Could you check a few things on this model? Use its own coordinates, in mm. Face numbers are marked on the shaded views. A direction names the side the tool comes from. Coordinates: 2 decimals unless noted, no trailing zeros. Order: outer loops, then holes, each group sorted by start corner. A loop starts at its lowest first (then second) coordinate and runs counter-clockwise, first axis right, second up. Notation, with made-up numbers: (6.25, 63) -> (41.25, 63) arc R25 ccw to (41.25, 101) -> close; hole circle Ø8 at (3.5, 87). An arc over 180 degrees is marked (long way). Use a Markdown table: item, result. Add a question column.
1) Thinking about a two-plate mould opening in Z: for the marked faces 1, 2 and 3, which applies, +Z half, -Z half, draft (parallel to the pull), parting line (faces both ways), or undercut?
2) If I drill on L1, parallel to Y at x = 5.5, z = -1; L2, parallel to Z at x = -2.5, y = 0.5; L3, parallel to X at y = 3.15, z = -18.5, over which ranges is the centre line in solid material (lowest first)? Write a range as [from, to].
3) If we section it at D-D (x = 5): Write out the boundary of the cut face in (y, z).
4) Which directions (+Z, -Z, +X, -X, +Y, -Y) give clear straight access to the entire face, cutting with the end or side of a thin tool? Please do the marked faces 4, 5 and 6.
5) If we section it at C-C (y = 3.3): Write out the boundary of the cut face in (x, z).
6) Will these pins go through, and if not, where does the flat tip stop? pin 1 Ø2 at (x, z) = (-1.5, -2.5) entering from +Y; pin 2 Ø6 at (x, z) = (4.5, -13) entering from +Y; pin 3 Ø1.5 at (x, y) = (1.5, 2.5) entering from +Z.
```python
from build123d import *

# Parameters (mm, degrees)
SM_BASE_FLANGE_1_DEPTH = 0.1
SKETCH_6_W             = 12.5
SKETCH_6_H             = 4
EXTRUDE_1_DEPTH        = 0.1
SKETCH_7_W             = 8.5
SKETCH_7_H             = 8.5
EXTRUDE_2_DEPTH        = 0.1
SKETCH_8_W             = 8.5
SKETCH_8_H             = 8.5
EXTRUDE_3_DEPTH        = 5.07
SKETCH_9_R             = 3
CUT_EXTRUDE_1_DEPTH    = 0.2
FILLET_2_R             = 0.5
FILLET_3_R             = 0.2
SKETCH_11_R            = 0.25
SKETCH_11_W            = 0.4
SKETCH_11_H            = 0.1
SKETCH_11_W_2          = 0.428641975
CUT_EXTRUDE_2_DEPTH    = 0.05
FILLET_4_R             = 0.2
FILLET_5_R             = 0.2
SKETCH_13_R            = 0.75
CUT_EXTRUDE_3_DEPTH    = 0.05
DOME_1_FACE_RADIUS     = 0.75
DOME_1_HEIGHT          = 0.1
CUT_EXTRUDE_4_DEPTH    = 0.05


# Sheet-metal steps are written as plain solids
with BuildPart() as part:
    # Sketch 1 → Базовая кромка1 (new body)
    with BuildSketch(Plane(origin=(0, 0, 0), x_dir=(1, 0, 0), z_dir=(0, 1, 0))):
        Polygon((-6.25, 4), (-6.25, 0), (6.25, 0), (6.25, 4), (3.3, 4), (3.3, 12.5), (4.25, 12.5), (4.25, 21), (-4.25, 21), (-4.25, 12.5), (-3.3, 12.5), (-3.3, 4), align=None)
    extrude(amount=-SM_BASE_FLANGE_1_DEPTH)

    # Эскиз6 → Бобышка-Вытянуть1 (add)
    with BuildSketch(Plane(origin=(0, 0, 0), x_dir=(1, 0, 0), z_dir=(0, 1, 0))):
        with Locations((0, 2)):
            Rectangle(SKETCH_6_W, SKETCH_6_H)
    extrude(amount=EXTRUDE_1_DEPTH)

    # Эскиз7 → Бобышка-Вытянуть2 (add)
    with BuildSketch(Plane.XZ.offset(0.1)):
        with Locations((0, -16.75)):
            Rectangle(SKETCH_7_W, SKETCH_7_H)
    extrude(amount=EXTRUDE_2_DEPTH)

    # Эскиз8 → Бобышка-Вытянуть3 (add)
    with BuildSketch(Plane(origin=(0, 0, 0), x_dir=(1, 0, 0), z_dir=(0, 1, 0))):
        with Locations((0, 16.75)):
            Rectangle(SKETCH_8_W, SKETCH_8_H)
    extrude(amount=EXTRUDE_3_DEPTH)

    # Эскиз9 → Вырез-Вытянуть1 (cut)
    with BuildSketch(Plane(origin=(0, 5.07, 0), x_dir=(1, 0, 0), z_dir=(0, 1, 0))):
        with Locations(Location((0, 16.75, 0), (0, 0, 270))):
            Circle(SKETCH_9_R)
    extrude(amount=-CUT_EXTRUDE_1_DEPTH, mode=Mode.SUBTRACT)

    # Скругление2
    fillet_2_edges = [part.edges().sort_by_distance(p)[0] for p in [
        (6.25, 0, -4),
        (-6.25, 0, -4),
    ]]
    fillet(fillet_2_edges, radius=FILLET_2_R)

    # Скругление3
    fillet_3_edges = [part.edges().sort_by_distance(p)[0] for p in [
        (6.25, 0, 0),
        (-6.25, 0, 0),
    ]]
    fillet(fillet_3_edges, radius=FILLET_3_R)

    # Эскиз11 → Вырез-Вытянуть2 (cut)
    with BuildSketch(Plane(origin=(0, 5.07, 0), x_dir=(1, 0, 0), z_dir=(0, 1, 0))):
        with Locations(Location((-2.504881476, 20.140788589, 0), (0, 0, 270))):
            Circle(SKETCH_11_R)
        Polygon((-3.404881476, 20.490788589), (-3.404881476, 19.790788589), (-2.804881476, 20.140788589), align=None)
        with Locations((-3.704881476, 20.290788589)):
            Rectangle(SKETCH_11_W, SKETCH_11_H)
        with Locations((-3.704881477, 19.990788589)):
            Rectangle(SKETCH_11_W_2, SKETCH_11_H)
    extrude(amount=-CUT_EXTRUDE_2_DEPTH, mode=Mode.SUBTRACT)

    # Скругление4
    fillet_4_edges = [part.edges().sort_by_distance(p)[0] for p in [
        (-4.25, 2.435, -12.5),
        (-4.25, 2.435, -21),
        (4.25, 2.435, -21),
        (4.25, 2.435, -12.5),
    ]]
    fillet(fillet_4_edges, radius=FILLET_4_R)

    # Скругление5
    fillet_5_edges = [part.edges().sort_by_distance(p)[0] for p in [
        (0, 5.07, -21),
        (-4.25, 5.07, -16.75),
        (0, 5.07, -12.5),
        (4.25, 5.07, -16.75),
        (4.191421356, 5.07, -12.558578644),
        (-4.191421356, 5.07, -12.558578644),
        (4.191421356, 5.07, -20.941421356),
        (-4.191421356, 5.07, -20.941421356),
    ]]
    fillet(fillet_5_edges, radius=FILLET_5_R)

    # Эскиз13 → Вырез-Вытянуть3 (cut)
    with BuildSketch(Plane(origin=(0, 4.87, 0), x_dir=(1, 0, 0), z_dir=(0, 1, 0))):
        with Locations(Location((0, 16.75, 0), (0, 0, 270))):
            Circle(SKETCH_13_R)
    extrude(amount=-CUT_EXTRUDE_3_DEPTH, mode=Mode.SUBTRACT)

    # Купол1: a dome of height H over a round flat face of radius A is a cap of a sphere of radius (A * A + H * H) / (2 * H)
    dome_1_r = (DOME_1_FACE_RADIUS * DOME_1_FACE_RADIUS + DOME_1_HEIGHT * DOME_1_HEIGHT) / (2 * DOME_1_HEIGHT)
    dome_1_base = Plane((0, 4.82, -16.75), z_dir=(0, 1, 0))
    with Locations(dome_1_base.offset(DOME_1_HEIGHT - dome_1_r)):
        dome_1_ball = Sphere(dome_1_r, mode=Mode.PRIVATE)
    add(split(dome_1_ball, bisect_by=dome_1_base, keep=Keep.TOP, mode=Mode.PRIVATE))

    # Эскиз14 → Вырез-Вытянуть4 (cut)
    with BuildSketch(Plane.XZ.offset(0.1)):
        with BuildLine():
            add(Edge.make_bspline(
                [(-6.003383397, -0.314306436), (-6.003208457, -0.309686598), (-6.002887878, -0.301220725), (-6.001492735, -0.289495252), (-5.998110788, -0.280222293), (-5.994627409, -0.272683421), (-5.990132541, -0.267041234), (-5.984854454, -0.263323548), (-5.979244173, -0.261024904), (-5.975355275, -0.260713676), (-5.973471862, -0.260562946)],
                knots=[0, 0, 0, 0, 1.628349121, 2.98395659, 4.129704748, 5.086564407, 5.897483759, 6.63370628, 7.338296972, 8, 8, 8, 8], degree=3))
            Line((-5.973471862, -0.260562946), (-5.410745912, -0.260562946))
            add(Edge.make_bspline(
                [(-5.410745912, -0.260562946), (-5.40885651, -0.260694679), (-5.405106012, -0.26095617), (-5.399775012, -0.263392441), (-5.394773829, -0.267176005), (-5.390117693, -0.272704247), (-5.385920232, -0.280035282), (-5.383175234, -0.289598664), (-5.381181748, -0.301173725), (-5.380956895, -0.309674519), (-5.380834377, -0.314306436)],
                knots=[0, 0, 0, 0, 0.664614152, 1.319270975, 2.035609743, 2.868536476, 3.856564754, 4.99840066, 6.364487051, 8, 8, 8, 8], degree=3))
            add(Edge.make_bspline(
                [(-5.380834377, -0.314306436), (-5.380864917, -0.318693721), (-5.380922402, -0.326951838), (-5.382944792, -0.338274401), (-5.385655893, -0.347798587), (-5.388864391, -0.35564771), (-5.393178768, -0.361704746), (-5.397996026, -0.366346051), (-5.403899926, -0.368834535), (-5.407971139, -0.369283488), (-5.410016362, -0.369509025)],
                knots=[0, 0, 0, 0, 1.527993431, 2.876117242, 3.994749226, 4.982414938, 5.814060196, 6.574910721, 7.284088933, 8, 8, 8, 8], degree=3))
            Line((-5.410016362, -0.369509025), (-5.629853985, -0.369509025))
            Line((-5.629853985, -0.369509025), (-5.629853985, -1.163259025))
            Line((-5.629853985, -1.163259025), (-5.429714202, -1.038749221))
            add(Edge.make_bspline(
                [(-5.429714202, -1.038749221), (-5.425149481, -1.036424176), (-5.417333568, -1.032443135), (-5.40641212, -1.02878606), (-5.397209622, -1.028178755), (-5.389825008, -1.032459821), (-5.384765717, -1.040366747), (-5.38236471, -1.05167421), (-5.38104661, -1.066189675), (-5.380910144, -1.077004214), (-5.380834377, -1.083008565)],
                knots=[0, 0, 0, 0, 1.300400407, 2.226601497, 2.927610547, 3.564433773, 4.290758113, 5.250986372, 6.473717283, 8, 8, 8, 8], degree=3))
            add(Edge.make_bspline(
                [(-5.380834377, -1.083008565), (-5.380843974, -1.08746989), (-5.380861627, -1.095675966), (-5.381887136, -1.106960532), (-5.38325169, -1.116425903), (-5.385371952, -1.124314191), (-5.388422962, -1.13096114), (-5.392349709, -1.136754986), (-5.397873467, -1.141735037), (-5.401965467, -1.144813428), (-5.404179965, -1.146479383)],
                knots=[0, 0, 0, 0, 1.503218099, 2.764990822, 3.816270798, 4.724653119, 5.507171343, 6.272807373, 7.065282303, 8, 8, 8, 8], degree=3))
            Line((-5.404179965, -1.146479383), (-5.642985878, -1.308682585))
            add(Edge.make_bspline(
                [(-5.642985878, -1.308682585), (-5.644337471, -1.309545988), (-5.647229049, -1.311393143), (-5.652486271, -1.313205889), (-5.658748264, -1.314930023), (-5.666283445, -1.316627774), (-5.675194902, -1.318142504), (-5.685696762, -1.318759354), (-5.698186972, -1.318943259), (-5.707267063, -1.318913018), (-5.712293093, -1.318896279)],
                knots=[0, 0, 0, 0, 0.541215428, 1.157868723, 1.870271028, 2.742350482, 3.770919716, 4.926365934, 6.298675888, 8, 8, 8, 8], degree=3))
            add(Edge.make_bspline(
                [(-5.712293093, -1.318896279), (-5.719020011, -1.318761234), (-5.731266064, -1.318515389), (-5.747870516, -1.317817694), (-5.761037615, -1.315832622), (-5.771126699, -1.313415241), (-5.77827598, -1.310034132), (-5.783062441, -1.30596597), (-5.784970741, -1.30095795), (-5.785318853, -1.297666831), (-5.78549124, -1.296037058)],
                knots=[0, 0, 0, 0, 1.938222078, 3.528446385, 4.779762996, 5.770770152, 6.501593536, 7.046594974, 7.527870594, 8, 8, 8, 8], degree=3))
            Line((-5.78549124, -1.296037058), (-5.78549124, -0.369509025))
            Line((-5.78549124, -0.369509025), (-5.974444595, -0.369509025))
            add(Edge.make_bspline(
                [(-5.974444595, -0.369509025), (-5.976483759, -0.369264404), (-5.980691588, -0.368759627), (-5.986880194, -0.366432009), (-5.991996556, -0.361778766), (-5.996351899, -0.35568764), (-5.99925034, -0.347770297), (-6.001822213, -0.338280185), (-6.003127762, -0.326904664), (-6.003294537, -0.318685637), (-6.003383397, -0.314306436)],
                knots=[0, 0, 0, 0, 0.711765533, 1.468732524, 2.24630102, 3.073130576, 4.044150543, 5.148818068, 6.480854525, 8, 8, 8, 8], degree=3))
        make_face()
    extrude(amount=-CUT_EXTRUDE_4_DEPTH, mode=Mode.SUBTRACT)


solid = part.part
```
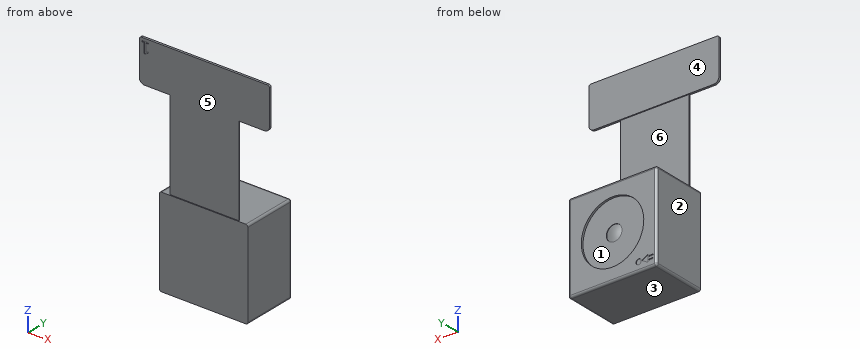
Answer sheet:
| question | item | result |
|---|---|---|
| 1 | face 1 | undercut |
| 1 | face 2 | draft |
| 1 | face 3 | -Z half |
| 2 | L1 | [-0.1, 0.1] |
| 2 | L2 | [-21, -12.5] |
| 2 | L3 | [-4.25, 4.25] |
| 3 | outline | (-0.1, -4) -> (0.1, -4) -> (0.1, 0) -> (-0.1, 0) -> close |
| 4 | face 4 | +Z, +X, -X, +Y |
| 4 | face 5 | +Z, +X, -X, -Y |
| 4 | face 6 | +X, -X, +Y |
| 5 | outline | (-4.25, -20.8) arc R0.2 ccw to (-4.05, -21) -> (4.05, -21) arc R0.2 ccw to (4.25, -20.8) -> (4.25, -12.7) arc R0.2 ccw to (4.05, -12.5) -> (-4.05, -12.5) arc R0.2 ccw to (-4.25, -12.7) -> close |
| 6 | pin 1 | y = 0.1 |
| 6 | pin 2 | y = 5.07 |
| 6 | pin 3 | z = -12.5 |
